Here's how the part is built. I have some questions about the finished solid (model axes, mm). Face numbers are marked on the shaded views. A direction names the side the tool comes from. Give positions to 0.01 mm unless a question says otherwise; leave off trailing zeros. Return JSON: item names as keys, results as strings. Group by question number.
(1) For P1, Ø1.1, axis at y = 15.5, z = -27.5, coming from the +X side; P2, Ø2, axis at x = 91.5, z = -11.5, coming from the +Y side; P3, Ø5.5, axis at y = 15, z = -15.5, coming from the +X side, each with a flat end and sliding along its axis, tell me the tip position at first contact or that it passes through.
(2) I need wall thicknesses on probe 1 along X at (y, z) = (2.45, -57); probe 2 along Z at (x, y) = (92.2, 23.6); probe 3 along Z at (x, y) = (92.2, 23.2). Which ranges of each line are inside material? Lowest first, please. Write a range as [from, to].
(3) If we section it at A-A (x = 99): State how many separate pieces and enclosed holes the cut face has, then the cut area to 3 significant figures.
(4) On a 3-axis mill with a long thin cutter (end or side, diameter ignored), from which of +Z, -Z, +X, -X, +Y, -Y can I reach the whole of each face in a straight line? I mean the marked faces 1 and 2. Say none if no direction works.
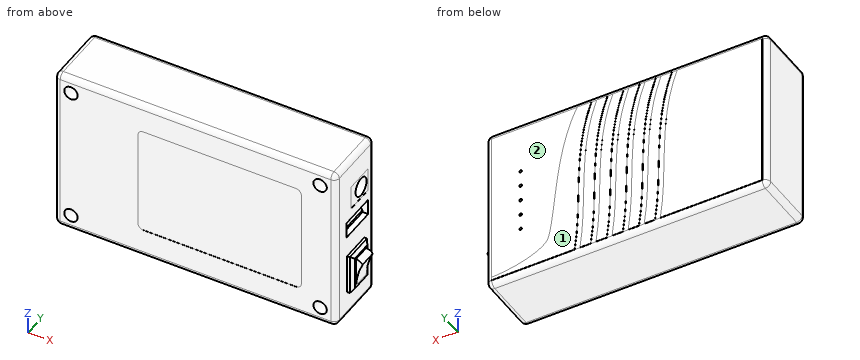
```python
from build123d import *
from OCP.BRepFilletAPI import BRepFilletAPI_MakeChamfer

# Parameters (mm, degrees)
SKETCH2_W           = 105
SKETCH2_H           = 63
BOSS_EXTRUDE1_DEPTH = 24
SKETCH3_W           = 9
SKETCH3_H           = 11
CUT_EXTRUDE1_DEPTH  = 0.05
SKETCH3_3_W         = 6
SKETCH3_3_H         = 14
CUT_EXTRUDE2_DEPTH  = 11
SKETCH3_4_W         = 15
SKETCH3_4_H         = 11
BOSS_EXTRUDE2_DEPTH = 1
SKETCH6_W           = 11
SKETCH6_H           = 6.5
BOSS_EXTRUDE3_DEPTH = 2.5
CUT_EXTRUDE3_DEPTH  = 128.188098893
FILLET1_R           = 2
SKETCH9_R           = 3.5
CUT_EXTRUDE4_DEPTH  = 10
BOSS_EXTRUDE4_DEPTH = 0.1
SKETCH11_R          = 0.5
CUT_EXTRUDE5_DEPTH  = 1
SKETCH12_R          = 2.5
CUT_EXTRUDE6_DEPTH  = 5
CUT_EXTRUDE7_DEPTH  = 0.05
SKETCH14_R          = 0.75
BOSS_EXTRUDE5_DEPTH = 8
FILLET2_R           = 0.75
SKETCH15_W          = 2
SKETCH15_H          = 11
BOSS_EXTRUDE6_DEPTH = 10
CHAMFER2_SIZE       = 0.9
CHAMFER2_SIZE2      = 0.519615242


with BuildPart() as part:
    # Sketch2 → Boss-Extrude1 (new body)
    with BuildSketch(Plane(origin=(0, 0, 0), x_dir=(1, 0, 0), z_dir=(0, 1, 0))):
        with Locations((52.5, 31.5)):
            Rectangle(SKETCH2_W, SKETCH2_H)
    extrude(amount=BOSS_EXTRUDE1_DEPTH)

    # Sketch3 → Cut-Extrude1 (cut)
    with BuildSketch(Plane(origin=(105, 0, 0), x_dir=(0, 0, -1), z_dir=(1, 0, 0))):
        with Locations((15.5, 15)):
            Rectangle(SKETCH3_W, SKETCH3_H)
    extrude(amount=-CUT_EXTRUDE1_DEPTH, mode=Mode.SUBTRACT)

    # Sketch3_3 → Cut-Extrude2 (cut)
    with BuildSketch(Plane(origin=(105, 0, 0), x_dir=(0, 0, -1), z_dir=(1, 0, 0))):
        with Locations((27, 13.5)):
            Rectangle(SKETCH3_3_W, SKETCH3_3_H)
    extrude(amount=-CUT_EXTRUDE2_DEPTH, mode=Mode.SUBTRACT)

    # Sketch3_4 → Boss-Extrude2 (add)
    with BuildSketch(Plane(origin=(105, 0, 0), x_dir=(0, 0, -1), z_dir=(1, 0, 0))):
        with Locations((45.5, 12.5)):
            Rectangle(SKETCH3_4_W, SKETCH3_4_H)
    extrude(amount=BOSS_EXTRUDE2_DEPTH)

    # Sketch5 → section 1 of loft3
    with BuildSketch(Plane(origin=(107, 0, 0), x_dir=(0, 0, -1), z_dir=(1, 0, 0)), mode=Mode.PRIVATE) as loft3_s1:
        with BuildLine():
            Line((39.25, 16.5), (51.75, 16.5))
            Line((51.75, 16.5), (51.75, 8.5))
            Line((51.75, 8.5), (39.25, 8.5))
            Line((39.25, 8.5), (39.25, 16.5))
        make_face()
    # loft from a face of the part (loft3)
    loft([part.faces().sort_by_distance((106, 12.5, -45.5))[0], loft3_s1.sketch])

    # Sketch6 → Boss-Extrude3 (add)
    with BuildSketch(Plane(origin=(107, 0, 0), x_dir=(0, 0, -1), z_dir=(1, 0, 0))):
        with Locations((45.5, 12.5)):
            Rectangle(SKETCH6_W, SKETCH6_H)
    extrude(amount=BOSS_EXTRUDE3_DEPTH)

    # Sketch8 → Cut-Extrude3 (cut, through all)
    with BuildSketch(Plane.XZ.offset(-9.25)):
        with BuildLine():
            ThreePointArc((107, -40), (108.382080547, -40.360838905), (109.5, -41.25))
            Line((109.5, -41.25), (109.5, -40))
            Line((109.5, -40), (107, -40))
        make_face()
        with BuildLine():
            ThreePointArc((109.5, -41.25), (107.777815786, -46.003927125), (107, -51))
            Line((107, -51), (109.5, -51))
            Line((109.5, -51), (109.5, -41.25))
        make_face()
    extrude(amount=-CUT_EXTRUDE3_DEPTH, mode=Mode.SUBTRACT)

    # Fillet1
    fillet1_edges = [part.edges().sort_by_distance(p)[0] for p in [
        (105, 24, -31.5),
        (52.5, 24, -63),
        (0, 24, -31.5),
        (52.5, 0, -63),
        (105, 0, -31.5),
        (52.5, 0, 0),
        (0, 0, -31.5),
        (0, 12, -63),
        (105, 12, -63),
        (105, 12, 0),
        (0, 12, 0),
        (52.5, 24, 0),
    ]]
    fillet(fillet1_edges, radius=FILLET1_R)

    # Sketch9 → Cut-Extrude4 (cut)
    with BuildSketch(Plane(origin=(104.95, 0, 0), x_dir=(0, 0, -1), z_dir=(1, 0, 0))):
        with Locations((15.5, 16)):
            Circle(SKETCH9_R)
    extrude(amount=-CUT_EXTRUDE4_DEPTH, mode=Mode.SUBTRACT)

    # Sketch10 → Boss-Extrude4 (add)
    with BuildSketch(Plane(origin=(0, 24, 0), x_dir=(1, 0, 0), z_dir=(0, 1, 0))):
        with BuildLine():
            Line((70.970468754, 2), (65.707078079, 2))
            add(Edge.make_bspline(
                [(65.707078079, 2), (72.906626661, 21.087182454), (69.043655607, 41.350605764), (71.994633575, 61)],
                knots=[0, 0, 0, 0, 1, 1, 1, 1], degree=3))
            Line((71.994633575, 61), (103, 61))
            Line((103, 61), (103, 59.688500541))
            add(Edge.make_bspline(
                [(103, 59.688500541), (100.793179796, 59.937762049), (87.368628023, 58.597582123), (82.605231661, 53.422629971)],
                knots=[0, 0, 0, 0, 1, 1, 1, 1], degree=3))
            add(Edge.make_bspline(
                [(82.605231661, 53.422629971), (80.465377293, 51.676680645), (78.981797834, 35.060590702), (78.981797834, 17.158731894), (70.970468754, 2)],
                knots=[0, 0, 0, 0, 0, 1, 1, 1, 1, 1], degree=4))
        make_face()
        with BuildLine():
            Line((63.707078079, 2), (59.707078079, 2))
            add(Edge.make_bspline(
                [(59.707078079, 2), (66.906626661, 21.087182454), (63.043655607, 41.350605764), (65.994633575, 61)],
                knots=[0, 0, 0, 0, 1, 1, 1, 1], degree=3))
            Line((65.994633575, 61), (69.994633575, 61))
            add(Edge.make_bspline(
                [(63.707078079, 2), (70.906626661, 21.087182454), (67.043655607, 41.350605764), (69.994633575, 61)],
                knots=[0, 0, 0, 0, 1, 1, 1, 1], degree=3))
        make_face()
        with BuildLine():
            Line((63.994633575, 61), (59.994633575, 61))
            add(Edge.make_bspline(
                [(53.707078079, 2), (60.906626661, 21.087182454), (57.043655607, 41.350605764), (59.994633575, 61)],
                knots=[0, 0, 0, 0, 1, 1, 1, 1], degree=3))
            Line((53.707078079, 2), (57.707078079, 2))
            add(Edge.make_bspline(
                [(57.707078079, 2), (64.906626661, 21.087182454), (61.043655607, 41.350605764), (63.994633575, 61)],
                knots=[0, 0, 0, 0, 1, 1, 1, 1], degree=3))
        make_face()
        with BuildLine():
            Line((57.994633575, 61), (53.994633575, 61))
            add(Edge.make_bspline(
                [(47.707078079, 2), (54.906626661, 21.087182454), (51.043655607, 41.350605764), (53.994633575, 61)],
                knots=[0, 0, 0, 0, 1, 1, 1, 1], degree=3))
            Line((47.707078079, 2), (51.707078079, 2))
            add(Edge.make_bspline(
                [(51.707078079, 2), (58.906626661, 21.087182454), (55.043655607, 41.350605764), (57.994633575, 61)],
                knots=[0, 0, 0, 0, 1, 1, 1, 1], degree=3))
        make_face()
        with BuildLine():
            Line((51.994633575, 61), (47.994633575, 61))
            add(Edge.make_bspline(
                [(41.707078079, 2), (48.906626661, 21.087182454), (45.043655607, 41.350605764), (47.994633575, 61)],
                knots=[0, 0, 0, 0, 1, 1, 1, 1], degree=3))
            Line((41.707078079, 2), (45.707078079, 2))
            add(Edge.make_bspline(
                [(45.707078079, 2), (52.906626661, 21.087182454), (49.043655607, 41.350605764), (51.994633575, 61)],
                knots=[0, 0, 0, 0, 1, 1, 1, 1], degree=3))
        make_face()
        with BuildLine():
            Line((45.994633575, 61), (41.994633575, 61))
            add(Edge.make_bspline(
                [(35.707078079, 2), (42.906626661, 21.087182454), (39.043655607, 41.350605764), (41.994633575, 61)],
                knots=[0, 0, 0, 0, 1, 1, 1, 1], degree=3))
            Line((35.707078079, 2), (39.707078079, 2))
            add(Edge.make_bspline(
                [(39.707078079, 2), (46.906626661, 21.087182454), (43.043655607, 41.350605764), (45.994633575, 61)],
                knots=[0, 0, 0, 0, 1, 1, 1, 1], degree=3))
        make_face()
        with BuildLine():
            Line((33.707078079, 2), (2, 2))
            Line((2, 2), (2, 61))
            Line((2, 61), (39.994633575, 61))
            add(Edge.make_bspline(
                [(33.707078079, 2), (40.906626661, 21.087182454), (37.043655607, 41.350605764), (39.994633575, 61)],
                knots=[0, 0, 0, 0, 1, 1, 1, 1], degree=3))
        make_face()
    extrude(amount=BOSS_EXTRUDE4_DEPTH)

    # Sketch11 → Cut-Extrude5 (cut)
    with BuildSketch(Plane(origin=(0, 24, 0), x_dir=(1, 0, 0), z_dir=(0, 1, 0))):
        with Locations(Location((92.2, 20, 0), (0, 0, 270))):
            Circle(SKETCH11_R)
        with Locations(Location((92.2, 26, 0), (0, 0, 270))):
            Circle(SKETCH11_R)
        with Locations(Location((92.2, 32, 0), (0, 0, 270))):
            Circle(SKETCH11_R)
        with Locations(Location((92.2, 38, 0), (0, 0, 270))):
            Circle(SKETCH11_R)
        with Locations(Location((92.2, 44, 0), (0, 0, 270))):
            Circle(SKETCH11_R)
    extrude(amount=-CUT_EXTRUDE5_DEPTH, mode=Mode.SUBTRACT)

    # Sketch12 → Cut-Extrude6 (cut)
    with BuildSketch(Plane.XZ):
        with Locations(Location((99, -6, 0), (0, 0, 270))):
            Circle(SKETCH12_R)
        with Locations(Location((99, -57, 0), (0, 0, 270))):
            Circle(SKETCH12_R)
    cut_extrude6 = extrude(amount=-CUT_EXTRUDE6_DEPTH, mode=Mode.SUBTRACT)

    # Mirror1: Cut-Extrude6 across plane
    add(cut_extrude6.mirror(Plane(origin=(52.5, 0, 0), x_dir=(0, 0, 1), z_dir=(1, 0, 0))), mode=Mode.SUBTRACT)

    # Sketch13 → Cut-Extrude7 (cut)
    with BuildSketch(Plane.XZ):
        with BuildLine():
            Line((33, -11), (90, -11))
            ThreePointArc((90, -11), (91.414213562, -11.585786438), (92, -13))
            Line((92, -13), (92, -50))
            ThreePointArc((92, -50), (91.414213562, -51.414213562), (90, -52))
            Line((90, -52), (33, -52))
            ThreePointArc((33, -52), (31.585786438, -51.414213562), (31, -50))
            Line((31, -50), (31, -13))
            ThreePointArc((31, -13), (31.585786438, -11.585786438), (33, -11))
        make_face()
    extrude(amount=-CUT_EXTRUDE7_DEPTH, mode=Mode.SUBTRACT)

    # Sketch14 → Boss-Extrude5 (add)
    with BuildSketch(Plane(origin=(94.95, 0, 0), x_dir=(0, 0, -1), z_dir=(1, 0, 0))):
        with Locations((15.5, 16)):
            Circle(SKETCH14_R)
    extrude(amount=BOSS_EXTRUDE5_DEPTH)

    # Fillet2
    fillet2_edges = [part.edges().sort_by_distance(p)[0] for p in [
        (102.95, 16, -14.75),
    ]]
    fillet(fillet2_edges, radius=FILLET2_R)

    # Sketch15 → Boss-Extrude6 (add)
    with BuildSketch(Plane(origin=(94, 0, 0), x_dir=(0, 0, -1), z_dir=(1, 0, 0))):
        with Locations((27.8, 13.5)):
            Rectangle(SKETCH15_W, SKETCH15_H)
    extrude(amount=BOSS_EXTRUDE6_DEPTH)

    # Chamfer2: one chamfer whose edges measure the first distance from different faces: ONE call of the kernel's chamfer builder (chamfer() names one face for all edges)
    chamfer2_edges_1 = [part.edges().sort_by_distance(p)[0] for p in [
        (104, 13.5, -28.8),
    ]]
    chamfer2_side_1 = [part.faces().sort_by_distance(p)[0] for p in [
        (99, 13.5, -28.8),
    ]]
    chamfer2_edges_2 = [part.edges().sort_by_distance(p)[0] for p in [
        (104, 19, -27.8),
    ]]
    chamfer2_side_2 = [part.faces().sort_by_distance(p)[0] for p in [
        (99, 19, -27.8),
    ]]
    chamfer2_edges_3 = [part.edges().sort_by_distance(p)[0] for p in [
        (104, 13.5, -26.8),
    ]]
    chamfer2_side_3 = [part.faces().sort_by_distance(p)[0] for p in [
        (99, 13.5, -26.8),
    ]]
    chamfer2_edges_4 = [part.edges().sort_by_distance(p)[0] for p in [
        (104, 8, -27.8),
    ]]
    chamfer2_side_4 = [part.faces().sort_by_distance(p)[0] for p in [
        (99, 8, -27.8),
    ]]
    chamfer2 = BRepFilletAPI_MakeChamfer(part.part.solid().wrapped)
    for e in chamfer2_edges_1:
        chamfer2.Add(CHAMFER2_SIZE, CHAMFER2_SIZE2, e.wrapped, chamfer2_side_1[0].wrapped)  # the first distance lies on this face
    for e in chamfer2_edges_2:
        chamfer2.Add(CHAMFER2_SIZE, CHAMFER2_SIZE2, e.wrapped, chamfer2_side_2[0].wrapped)  # the first distance lies on this face
    for e in chamfer2_edges_3:
        chamfer2.Add(CHAMFER2_SIZE, CHAMFER2_SIZE2, e.wrapped, chamfer2_side_3[0].wrapped)  # the first distance lies on this face
    for e in chamfer2_edges_4:
        chamfer2.Add(CHAMFER2_SIZE, CHAMFER2_SIZE2, e.wrapped, chamfer2_side_4[0].wrapped)  # the first distance lies on this face
    add(Compound.cast(chamfer2.Shape()), mode=Mode.REPLACE)


solid = part.part
```
Values:
{
 "1": {"P1": "x = 104", "P2": "y = 24", "P3": "x = 104.95"},
 "2": {"probe 1": "[0, 3.5], [8.5, 96.5], [101.5, 105]", "probe 2": "[-62.2, -44.5], [-43.5, -38.5], [-37.5, -32.5], [-31.5, -26.5], [-25.5, -20.5], [-19.5, -0.8]", "probe 3": "[-62.6, -44.5], [-43.5, -38.5], [-37.5, -32.5], [-31.5, -26.5], [-25.5, -20.5], [-19.5, -0.4]"},
 "3": {"separate pieces": "3", "enclosed holes": "2", "area": "1,360 mm2"},
 "4": {"face 1": "+Z, -Z, +X, -X, +Y", "face 2": "+Z, +X, +Y"}
}
